from build123d import *

# Parameters (mm, degrees)
F0_W      = 16.1925
F0_H      = 15.875
F1_DEPTH  = 0.3175
F3_DEPTH  = 5.715
F5_DEPTH  = 0.79375
F6_R      = 0.79375
F7_DEPTH  = 0.79375
F8_DEPTH  = 0.3175
F9_W      = 1.5875
F9_H      = 0.635
F10_DEPTH = 1.5875
F11_DEPTH = 0.3175
F12_W     = 1.5875
F12_H     = 1.5875
F13_DEPTH = 0.79375
F14_DEPTH = 0.15875
F15_R     = 0.5
F16_DEPTH = 25.4
F17_R     = 1.5875
F18_DEPTH = 3.175


with BuildPart() as f1:
    # F0 (on Top) → F1 (new body)
    with BuildSketch(Plane.XY):
        Polygon((-25.671613648, 46.3675076752), (-18.369113648, 27.4050211887), (-18.369113648, 7.0850211887), (10.523386352, 7.0850211887), (10.523386352, 27.4050211887), (17.825886352, 46.3675076752), align=None)
        with Locations((-3.922863648, 20.1025211887)):
            Rectangle(F0_W, F0_H, mode=Mode.SUBTRACT)
    extrude(amount=F1_DEPTH)

    # F2 (on face) → F3 (join)
    with BuildSketch(Plane.XY.offset(0.3175)):
        Polygon((17.825886352, 46.3675076752), (17.032136352, 46.3675076752), (9.729636352, 27.4050211887), (9.729636352, 7.0850211887), (10.523386352, 7.0850211887), (10.523386352, 27.4050211887), align=None)
        Polygon((-24.877863648, 46.3675076752), (-25.671613648, 46.3675076752), (-18.369113648, 27.4050211887), (-18.369113648, 7.0850211887), (-17.575363648, 7.0850211887), (-17.575363648, 27.4050211887), align=None)
    extrude(amount=F3_DEPTH)

    # F4 (on face) → F5 (join)
    with BuildSketch(Plane.XY.offset(6.0325)):
        Polygon((-19.3472738705, 29.9450211887), (-18.369113648, 27.4050211887), (10.523386352, 27.4050211887), (11.5015465745, 29.9450211887), align=None)
    extrude(amount=F5_DEPTH)

    # F6 (on face) → F7 (cut)
    with BuildSketch(Plane.XY.offset(6.82625)):
        with Locations((-12.019113648, 28.6750211887)):
            Circle(F6_R)
        with Locations((4.173386352, 28.6750211887)):
            Circle(F6_R)
    extrude(amount=-F7_DEPTH, mode=Mode.SUBTRACT)

    # F8 (add): a face of the model
    f8_faces = [f1.faces().sort_by_distance(p)[0] for p in [
        (-3.922863648, 30.216271867, 0),
    ]]
    extrude(f8_faces, amount=F8_DEPTH)

    # F9 (on face) → F10 (join)
    with BuildSketch(Plane.XZ.offset(-7.0850211887)):
        Polygon((-17.575363648, 0.3175), (-18.369113648, 0.3175), (-18.369113648, -0.3175), (-16.781613648, -0.3175), (-16.781613648, 0.3175), align=None)
        with Locations((-14.400363648, 0)):
            Rectangle(F9_W, F9_H)
        with Locations((1.379386352, 0)):
            Rectangle(F9_W, F9_H)
        with Locations((4.554386352, 0)):
            Rectangle(F9_W, F9_H)
    extrude(amount=F10_DEPTH)

    # F11 (add): a face of the model
    f11_faces = [f1.faces().sort_by_distance(p)[0] for p in [
        (-3.9482759262, 29.9813117116, -0.3175),
    ]]
    extrude(f11_faces, amount=F11_DEPTH)

    # F12 (on face) → F13 (join)
    with BuildSketch(Plane.XY.offset(0.3175)):
        with Locations((-17.575363648, 6.2912711887)):
            Rectangle(F12_W, F12_H)
        with Locations((-14.400363648, 6.2912711887)):
            Rectangle(F12_W, F12_H)
        with Locations((1.379386352, 6.2912711887)):
            Rectangle(F12_W, F12_H)
        with Locations((4.554386352, 6.2912711887)):
            Rectangle(F12_W, F12_H)
    extrude(amount=F13_DEPTH)

    # F14 (cut): a face of the model
    f14_faces = [f1.faces().sort_by_distance(p)[0] for p in [
        (-3.9482759262, 29.9813117116, -0.635),
    ]]
    extrude(f14_faces, amount=-F14_DEPTH, mode=Mode.SUBTRACT)

    # F15 (on face) → F16 (cut)
    with BuildSketch(Plane(origin=(-18.369113648, 0, 0), x_dir=(0, -1, 0), z_dir=(-1, 0, 0))):
        with Locations((-6.2912711887, 0.3175)):
            Circle(F15_R)
    extrude(amount=-F16_DEPTH, mode=Mode.SUBTRACT)

    # F17 (on face) → F18 (join)
    with BuildSketch(Plane(origin=(0, 0, -0.47625), x_dir=(1, 0, 0), z_dir=(0, 0, -1))):
        with Locations((-15.194113648, -28.0400211887)):
            Circle(F17_R)
        with Locations((7.348386352, -28.0400211887)):
            Circle(F17_R)
    extrude(amount=F18_DEPTH)


solid = f1.part
For this review, take the finished solid that the model builds, in its own axes (mm). Give positions to 0.01 mm unless a question says otherwise; leave off trailing zeros. Loops run counter-clockwise (first coordinate to the right, second up) from the corner with the lowest first, then second, coordinate; pieces in that order, holes last. Notation, with made-up numbers: M 49.25,38 L 72.25,38 A21 ccw 72.25,42 Z; hole C 30.25,7.25 d11. An arc over 180 degrees is marked long. Put each result on its own line as item: value. Start each with the question number.
(1) Add section A-A, the plane x = -9. Write out the cut boundary in (y, z).
(2) Add section C-C, the plane z = 2.5. Write out the cut boundary in (x, y), then the cut area to 3 significant figures.
(3) Wall thickness on L1, parallel to Z at x = 4.5, y = 27.5; L2, parallel to X at y = 15, z = 5.25; L3, parallel to X at y = 19, z = 0: over which ranges is each line inside the solid? List them lowest first.
(4) Add section D-D, the plane y = 41.5. Write out the cut boundary in (x, z).
(5) For pin 1 (2 mm diameter, centred on y = 18.5, z = 1.5, fed in from +X); pin 2 (1.5 mm diameter, centred on x = 0.5, y = 41, fed in from -Z); pin 3 (1.7 mm diameter, centred on x = 1.5, y = 6, fed in from +Z), all flat-tipped, find the tip position at first contact; note any pin that passes through.
(6) The part is to be moulded in two halves that separate along X. For faces 1 (the flat face through (-17.575, 17, 3)), 2 (the flat face through (-21.175, 36.754, 3.135)), 3 (the flat face through (10.523, 17, 3)), 4 (the flat face through (7, 28, -3.651)), say which applies: +X half, -X half, draft (parallel to the pull), parting line (faces both ways), or undercut.
(7) Add section B-B, the plane y = 16. Write out the cut boundary in (x, z), then the cut area to 3 significant figures.
Result:
1. outline: M 7.09,-0.48 L 12.17,-0.48 L 12.17,0.32 L 7.09,0.32 Z; M 27.41,6.03 L 29.95,6.03 L 29.95,6.83 L 27.41,6.83 Z; M 28.04,-0.48 L 46.37,-0.48 L 46.37,0.32 L 28.04,0.32 Z
2. outline: M -25.67,46.37 L -18.37,27.41 L -18.37,7.09 L -17.58,7.09 L -17.58,27.41 L -24.88,46.37 Z; M 9.73,7.09 L 10.52,7.09 L 10.52,27.41 L 17.83,46.37 L 17.03,46.37 L 9.73,27.41 Z
2. area: 62.4 mm^2
3. L1: z = -0.48 to 0.32, 6.03 to 6.83
3. L2: x = -18.37 to -17.58, 9.73 to 10.52
3. L3: x = -18.37 to -12.02, 4.17 to 10.52
4. outline: M -23.8,-0.48 L 15.95,-0.48 L 15.95,6.03 L 15.16,6.03 L 15.16,0.32 L -23,0.32 L -23,6.03 L -23.8,6.03 Z
5. pin 1: stops at x = 10.52
5. pin 2: stops at z = -0.48
5. pin 3: stops at z = 1.11
6. face 1: undercut
6. face 2: undercut
6. face 3: +X half
6. face 4: draft
7. outline: M -18.37,-0.48 L -12.02,-0.48 L -12.02,0.32 L -17.58,0.32 L -17.58,6.03 L -18.37,6.03 Z; M 4.17,-0.48 L 10.52,-0.48 L 10.52,6.03 L 9.73,6.03 L 9.73,0.32 L 4.17,0.32 Z
7. area: 19.2 mm^2
